from build123d import *

# Parameters (mm, degrees)
F0_R     = 50.8
F0_R_2   = 6.35
F0_R_3   = 19.05
F1_DEPTH = 12.7
F2_R     = 25.4
F3_DEPTH = 38.1


with BuildPart() as f1:
    # F0 (on Right) → F1 (new body)
    with BuildSketch(Plane.YZ):
        Circle(F0_R)
        with Locations((-28.575, -28.575)):
            Circle(F0_R_2, mode=Mode.SUBTRACT)
        Circle(F0_R_3, mode=Mode.SUBTRACT)
        with Locations((28.575, -28.575)):
            Circle(F0_R_2, mode=Mode.SUBTRACT)
        with Locations((-28.575, 28.575)):
            Circle(F0_R_2, mode=Mode.SUBTRACT)
        with Locations((28.575, 28.575)):
            Circle(F0_R_2, mode=Mode.SUBTRACT)
    extrude(amount=F1_DEPTH)

    # F2 (on Right) → F3 (join)
    with BuildSketch(Plane.YZ):
        Circle(F2_R)
    extrude(amount=F3_DEPTH)

    # F4: F1 across face


with BuildPart() as f1_1:
    add(f1.part)
    add(f1.part.mirror(Plane.YZ.offset(38.1)))


solid = f1_1.part
Design review of the part built by this model. Coordinates are the model's own, in mm. A direction names the side the tool comes from. Round coordinates to 2 decimals unless told otherwise and drop trailing zeros. Write each loop counter-clockwise with the first axis right and the second up, starting at its lowest first coordinate (ties: lowest second). Pieces come first, ordered by that corner, then holes. Notation, with made-up numbers: M 76,61.5 L 124,61.5 A35 ccw 124,99.5 Z; hole C 67,-11.75 d10. An arc over 180 degrees is marked long. One line per item, written item: value. Start each with the question number.
1. Take a section at B-B on z = 0. State the section outline as (x, y) points, then the cut area to 3 significant figures.
2. Take a section at A-A on y = -33.5. State the section outline as (x, z) points.
3. To check wall thickness, follow probe 1 along X at (y, z) = (18, 37); probe 2 along Z at (x, y) = (5, -34); probe 3 along Z at (x, y) = (71, -25). State the ranges of each line that lie inside material, in increasing order. Write a range as from..to.
4. Clearance check with flat-ended pins moving along their axes: P1, Ø14.5, axis at y = -28.575, z = -28.575, coming from the -X side; P2, Ø7.5, axis at y = -28.575, z = 28.575, coming from the +X side; P3, Ø5, axis at x = 65, y = -19.5, coming from the -Z side; P4, Ø12, axis at x = 57, z = -15.5, coming from the +Y side. State where each tip first meets the part, or that it passes through.
5. Draft analysis for pull direction Z (two halves, no side actions). For faces 3 (the face through (12.7, 10.6, 23.3)), 4 (the face through (6.261, -11.012, -49.592)), 5 (the face through (69.94, -22.71, 26.14)), 6 (the face through (6.261, -22.518, -26.668)), state which applies: pulls with the +Z half, pulls with the -Z half, needs draft (parallel to the pull), parting line crosses it, or undercut.
6. For faces 1 (the face through (6.261, 23.895, -24.283)), 2 (the face through (38.456, -5.506, -24.796)), list the 3-axis set-ups (+Z, -Z, +X, -X, +Y, -Y) from which the entire face can be reached by the end or side of a thin tool; tool diameter is ignored.
7. Take a section at D-D on x = 9. State the section outline as (y, z) points (3 decimals).
Computed:
1. outline: M 0,-50.8 L 12.7,-50.8 L 12.7,-25.4 L 63.5,-25.4 L 63.5,-50.8 L 76.2,-50.8 L 76.2,50.8 L 63.5,50.8 L 63.5,25.4 L 12.7,25.4 L 12.7,50.8 L 0,50.8 Z
1. area: 5,160 mm²
2. outline: M 0,-38.19 L 12.7,-38.19 L 12.7,-32.58 L 0,-32.58 Z; M 0,-24.57 L 12.7,-24.57 L 12.7,24.57 L 0,24.57 Z; M 0,32.58 L 12.7,32.58 L 12.7,38.19 L 0,38.19 Z; M 63.5,-38.19 L 76.2,-38.19 L 76.2,-32.58 L 63.5,-32.58 Z; M 63.5,-24.57 L 76.2,-24.57 L 76.2,24.57 L 63.5,24.57 Z; M 63.5,32.58 L 76.2,32.58 L 76.2,38.19 L 63.5,38.19 Z
3. probe 1: x = 0..12.7, 63.5..76.2
3. probe 2: z = -37.74..-31.88, -25.27..25.27, 31.88..37.74
3. probe 3: z = -44.22..-33.82, -23.33..23.33, 33.82..44.22
4. P1: stops at x = 0
4. P2: passes through
4. P3: stops at z = -47.87
4. P4: stops at y = 23.56
5. face 3: needs draft
5. face 4: parting line crosses it
5. face 5: undercut
5. face 6: undercut
6. face 1: +X, -X
6. face 2: none
7. outline: C 0,0 d101.6; hole C -28.575,-28.575 d12.7; hole C -28.575,28.575 d12.7; hole C 28.575,-28.575 d12.7; hole C 28.575,28.575 d12.7
